```python
from build123d import *

# Parameters (mm, degrees)
F1_DEPTH      = 40
F1_DEPTH_BACK = 40
F2_R          = 5
F3_R          = 39.99999
F4_R          = 10
F5_DEPTH      = 52.2
F7_DEPTH      = 25
F8_R          = 20


# Not quite as in the source:
# - a fillet or chamfer is up to 0.001 mm smaller than in the source, because OpenCascade refuses the exact size


with BuildPart() as f1:
    # F0 (on Top) → F1 (new body, two sides)
    with BuildSketch(Plane.XY) as f1_sk:
        Polygon((-44.4148934171, 0), (105.5851065829, 0), (105.5851065829, 10), (-4.0003745738, 10), (-49.7738772657, 89.2820323028), (-58.4341313035, 84.2820323028), (-28.4341313035, 32.3205080757), (-45.7546393792, 22.3205080757), (-75.7546393792, 74.2820323028), (-84.4148934171, 69.2820323028), align=None)
    extrude(amount=F1_DEPTH)
    extrude(f1_sk.sketch, amount=-F1_DEPTH_BACK)

    # F2
    f2_edges = [f1.edges().sort_by_distance(p)[0] for p in [
        (-4.000375, 10, 0),
    ]]
    fillet(f2_edges, radius=F2_R)

    # F3 (radius 40 in the source; OpenCascade refuses exactly that, so slightly less here)
    f3_edges = [f1.edges().sort_by_distance(p)[0] for p in [
        (-54.104004, 86.782032, 40),
        (-80.084766, 71.782032, 40),
        (-80.084766, 71.782032, -40),
        (-54.104004, 86.782032, -40),
    ]]
    fillet(f3_edges, radius=F3_R)

    # F4 (on face) → F5 (cut)
    with BuildSketch(Plane(origin=(1.3298460886, 0.7677869972, 0), x_dir=(-0.5, 0.8660254038, 0), z_dir=(0.8660254038, 0.5, 0))):
        with Locations((60.2471926707, 0)):
            Circle(F4_R)
    extrude(amount=-F5_DEPTH, mode=Mode.SUBTRACT)

    # F6 (on face) → F7 (cut)
    with BuildSketch(Plane(origin=(0, 10, 0), x_dir=(-1, 0, 0), z_dir=(0, 1, 0))):
        with BuildLine():
            ThreePointArc((-45.5851065829, -10), (-55.5851065829, 0), (-45.5851065829, 10))
            Line((-45.5851065829, 10), (-105.5851065829, 10))
            Line((-105.5851065829, 10), (-105.5851065829, -10))
            Line((-105.5851065829, -10), (-45.5851065829, -10))
        make_face()
        with BuildLine():
            ThreePointArc((-45.5851065829, -10), (-38.5140387711, -7.0710678119), (-35.5851065829, 0))
            ThreePointArc((-35.5851065829, 0), (-38.5140387711, 7.0710678119), (-45.5851065829, 10))
            ThreePointArc((-45.5851065829, 10), (-55.5851065829, 0), (-45.5851065829, -10))
        make_face()
    extrude(amount=-F7_DEPTH, mode=Mode.SUBTRACT)

    # F8
    f8_edges = [f1.edges().sort_by_distance(p)[0] for p in [
        (105.585107, 5, -40),
        (105.585107, 5, 40),
    ]]
    fillet(f8_edges, radius=F8_R)


solid = f1.part
```
Work out the finished part from the listing and answer in its coordinate system (mm). A direction names the side the tool comes from. Coordinates: 2 decimals unless noted, no trailing zeros. Write each loop counter-clockwise with the first axis right and the second up, starting at its lowest first coordinate (ties: lowest second). Pieces come first, ordered by that corner, then holes.
Q1. Which of the six approach directions +Z, -Z, +X, -X, +Y, -Y give full straight-line access (tool end or side, diameter ignored) to faces 1 (the face through (75, 5, 10)), 2 (the face through (-60.25, 27.43, -8.33)), 3 (the face through (-36.973, 27.391, 0.56))?
Q2. Find the intervals of material crossed by line 1 (Y direction, x = 58, z = 18.5); line 2 (X direction, y = 70.5, z = 13); line 3 (Y direction, x = -53.5, z = 18), in increasing order.
Q3. A cutting plane is placed at B-B, the plane z = -8. Give the vertices of the cut face in (x, y).
Q4. A cutting plane is placed at D-D, the plane z = -31. Give the vertices of the cut face in (x, y), then the cut area to 3 significant figures.
Q5. Determine the mould class of faces 4 (the face through (-6, 11, -40)), 5 (the face through (-74.131, 61.33, 28.594)), 6 (the face through (105.585, 5, -15)), 7 (the face through (-37.83, 58.74, 3)) for opening direction X: released by +X, released by -X, zero draft, split by the parting line, or undercut.
Q6. A cutting plane is placed at A-A, the plane x = 68.5. Give the vertices of the cut face in (y, z), then the cut area to 3 significant figures.
Q7. A cutting plane is placed at C-C, the plane y = 5.5. Give the vertices of the cut face in (x, z).
Q8. Each of these flat-tipped pins is pushed along its axis until it touches: pin 1 Ø6 at (y, z) = (71.5, -7.5) entering from -X; pin 2 Ø5 at (y, z) = (44, 17.5) entering from +X; pin 3 Ø3 at (y, z) = (35, -9.5) entering from -X. Where does it stop, or does it pass through?
Findings below:
1. face 1: +X, +Y, -Y
1. face 2: +Z, -Z, -X, -Y
1. face 3: +Z, -Z
2. line 1: y = 0 to 10
2. line 2: x = -77.96 to -73.57, -50.48 to -38.93
2. line 3: y = 15.74 to 35.74, 75.74 to 82.19
3. outline: (-84.01, 68.58) - (-66.43, 38.14) - (-57.77, 43.14) - (-75.35, 73.58) - close; (-60.43, 27.75) - (-44.41, 0) - (39.59, 0) - (39.59, 10) - (-1.11, 10) arc R5 cw to (-5.44, 12.5) - (-25.79, 47.75) - (-34.45, 42.75) - (-28.43, 32.32) - (-45.75, 22.32) - (-51.77, 32.75) - close; (-58.03, 83.58) - (-40.45, 53.14) - (-31.79, 58.14) - (-49.37, 88.58) - close
4. outline: (-77.05, 56.53) - (-44.41, 0) - (102.29, 0) - (102.29, 10) - (-1.11, 10) arc R5 cw to (-5.44, 12.5) - (-42.41, 76.53) - (-51.07, 71.53) - (-28.43, 32.32) - (-45.75, 22.32) - (-68.39, 61.53) - close
4. area: 3,200 mm2
5. face 4: zero draft
5. face 5: released by -X
5. face 6: released by +X
5. face 7: undercut
6. outline: (0, -40) - (10, -40) - (10, -10) - (0, -10) - close; (0, 10) - (10, 10) - (10, 40) - (0, 40) - close
6. area: 600 mm2
7. outline: (-47.59, -40) - (85.59, -40) arc R20 ccw to (105.59, -20) - (105.59, -10) - (45.59, -10) arc R10 cw to (45.59, 10) - (105.59, 10) - (105.59, 20) arc R20 ccw to (85.59, 40) - (-47.59, 40) - close
8. pin 1: stops at x = -84.19
8. pin 2: stops at x = -22.19
8. pin 3: stops at x = -65.49
